from build123d import *

# Parameters (mm, degrees)
ESBO_O1_W                                            = 25
ESBO_O1_H                                            = 14
RESSALTO_EXTRUS_O1_DEPTH                             = 4
ESBO_O2_W                                            = 4
ESBO_O2_H                                            = 14
RESSALTO_EXTRUS_O2_DEPTH                             = 5
ESBO_O4_W                                            = 25
ESBO_O4_H                                            = 2
CORTE_EXTRUS_O1_DEPTH                                = 31.033314835
ESCAREADO_PARA_PARAFUSO_COM_CABE_A_ESCAR_D           = 2.4
ESCAREADO_PARA_PARAFUSO_COM_CABE_A_ESCAR_DEPTH       = 15
ESCAREADO_PARA_PARAFUSO_COM_CABE_A_ESCAR_CSINK_D     = 4.4
ESCAREADO_PARA_PARAFUSO_COM_CABE_A_ESCAR_CSINK_ANGLE = 90
ESCAREADO_PARA_PARAFUSO_COM_CABE_A_ESCAR_TIP         = 0.721032743
FILETE1_R                                            = 2
CHANFRO1_SIZE                                        = 1


with BuildPart() as part:
    # Esboço1 → Ressalto-extrusão1 (new body)
    with BuildSketch(Plane.XY):
        with Locations((12.5, 7)):
            Rectangle(ESBO_O1_W, ESBO_O1_H)
    extrude(amount=RESSALTO_EXTRUS_O1_DEPTH)

    # Esboço2 → Ressalto-extrusão2 (add)
    with BuildSketch(Plane.XY.offset(4)):
        with Locations((23, 7)):
            Rectangle(ESBO_O2_W, ESBO_O2_H)
    extrude(amount=RESSALTO_EXTRUS_O2_DEPTH)

    # Esboço4 → Corte-extrusão1 (cut, through all)
    with BuildSketch(Plane.XY.offset(9)):
        with Locations((12.5, 13)):
            Rectangle(ESBO_O4_W, ESBO_O4_H)
        with Locations((12.5, 1)):
            Rectangle(ESBO_O4_W, ESBO_O4_H)
    extrude(amount=-CORTE_EXTRUS_O1_DEPTH, mode=Mode.SUBTRACT)

    # Escareado para parafuso com cabeça escareada chata de M21
    with Locations(Plane(origin=(21, 10, 7), x_dir=(0, -1, 0), z_dir=(-1, 0, 0))):
        with Locations((0, 0), (6, 0)):
            CounterSinkHole(ESCAREADO_PARA_PARAFUSO_COM_CABE_A_ESCAR_D / 2, ESCAREADO_PARA_PARAFUSO_COM_CABE_A_ESCAR_CSINK_D / 2, depth=ESCAREADO_PARA_PARAFUSO_COM_CABE_A_ESCAR_DEPTH, counter_sink_angle=ESCAREADO_PARA_PARAFUSO_COM_CABE_A_ESCAR_CSINK_ANGLE)
            with Locations((0, 0, -(ESCAREADO_PARA_PARAFUSO_COM_CABE_A_ESCAR_DEPTH + ESCAREADO_PARA_PARAFUSO_COM_CABE_A_ESCAR_TIP / 2))):  # 118° drill point
                Cone(0, ESCAREADO_PARA_PARAFUSO_COM_CABE_A_ESCAR_D / 2, ESCAREADO_PARA_PARAFUSO_COM_CABE_A_ESCAR_TIP, mode=Mode.SUBTRACT)

    # Filete1
    filete1_edges = [part.edges().sort_by_distance(p)[0] for p in [
        (25, 7, 0),
    ]]
    fillet(filete1_edges, radius=FILETE1_R)

    # Chanfro1
    # the kernel refuses this chamfer: 1 mm, written as the material it takes off along each edge
    with BuildSketch(Plane(origin=(0, 14.571682988, 4), x_dir=(-0.027495876610586365, 0, -0.9996219169112968), z_dir=(0, -1, 0))) as chanfro1_piece_1:
        Polygon((CHANFRO1_SIZE * 0.999621916911, CHANFRO1_SIZE * 0.0274958766106), (-CHANFRO1_SIZE * 0.0274958766106, CHANFRO1_SIZE * 0.999621916911), (0, 0), align=None)
    extrude(amount=15.143365976, mode=Mode.SUBTRACT)
    with BuildSketch(Plane(origin=(21, 12, 4), x_dir=(0, 0.02749587661058735, -0.9996219169112968), z_dir=(-1, 0, 0))) as chanfro1_piece_2:
        Polygon((CHANFRO1_SIZE * 0.999621916911, CHANFRO1_SIZE * 0.0274958766106), (-CHANFRO1_SIZE * 0.0274958766106, CHANFRO1_SIZE * 0.999621916911), (0, 0), align=None)
    extrude(amount=23.571682988, mode=Mode.SUBTRACT)
    with BuildSketch(Plane(origin=(21, 12, 5.344832151), x_dir=(0.9996219169112968, 0.027495876610585647, 0), z_dir=(0, 0, 1)), Plane(origin=(21, 2, 11.571682988), x_dir=(0.9996219169112968, -0.027495876610586726, 0), z_dir=(0, 0, -1))) as chanfro1_piece_3:
        Polygon((CHANFRO1_SIZE * 0.999621916911, -CHANFRO1_SIZE * 0.0274958766106), (-CHANFRO1_SIZE * 0.0274958766106, -CHANFRO1_SIZE * 0.999621916911), (0, 0), align=None)
    extrude(amount=6.226850837, mode=Mode.SUBTRACT)
    with BuildSketch(Plane(origin=(-2.571682988, 2, 4), x_dir=(0, 0.9996219169112968, 0.027495876610586487), z_dir=(1, 0, 0))) as chanfro1_piece_4:
        Polygon((CHANFRO1_SIZE * 0.999621916911, -CHANFRO1_SIZE * 0.0274958766106), (-CHANFRO1_SIZE * 0.0274958766106, -CHANFRO1_SIZE * 0.999621916911), (0, 0), align=None)
    extrude(amount=23.571682988, mode=Mode.SUBTRACT)
    with BuildSketch(Plane(origin=(21, 2, 8.655167849), x_dir=(-0.027495876610585623, 0.9996219169112968, 0), z_dir=(0, 0, -1))) as chanfro1_piece_5:
        Polygon((CHANFRO1_SIZE * 0.999621916911, CHANFRO1_SIZE * 0.0274958766106), (-CHANFRO1_SIZE * 0.0274958766106, CHANFRO1_SIZE * 0.999621916911), (0, 0), align=None)
    extrude(amount=4.655167849, mode=Mode.SUBTRACT)
    with BuildSketch(Plane(origin=(21, 12, 4), x_dir=(0.9996219169112968, 0.027495876610585647, 0), z_dir=(0, 0, 1))) as chanfro1_piece_6:
        Polygon((CHANFRO1_SIZE * 0.999621916911, -CHANFRO1_SIZE * 0.0274958766106), (-CHANFRO1_SIZE * 0.0274958766106, -CHANFRO1_SIZE * 0.999621916911), (0, 0), align=None)
    extrude(amount=4.655167849, mode=Mode.SUBTRACT)
    with BuildSketch(Plane(origin=(23.571682988, 12, 4), x_dir=(0, 0.027495876610585623, -0.9996219169112968), z_dir=(-1, 0, 0))) as chanfro1_piece_7a_section:
        Polygon((CHANFRO1_SIZE * 0.999621916911, CHANFRO1_SIZE * 0.0274958766106), (-CHANFRO1_SIZE * 0.0274958766106, CHANFRO1_SIZE * 0.999621916911), (0, 0), align=None)
    chanfro1_piece_7a = extrude(amount=26.143365976, mode=Mode.PRIVATE)
    chanfro1_piece_7a = split(chanfro1_piece_7a, bisect_by=Plane(origin=(21, 11.670206373, 3.670206373), z_dir=(1, 0, 0)), keep=Keep.TOP, mode=Mode.PRIVATE)
    with BuildSketch(Plane(origin=(21, 12, 1.428317012), x_dir=(0.9996219169112968, 0.027495876610585647, 0), z_dir=(0, 0, 1))) as chanfro1_piece_7b_section:
        Polygon((CHANFRO1_SIZE * 0.999621916911, -CHANFRO1_SIZE * 0.0274958766106), (-CHANFRO1_SIZE * 0.0274958766106, -CHANFRO1_SIZE * 0.999621916911), (0, 0), align=None)
    chanfro1_piece_7b = extrude(amount=7.226850837, mode=Mode.PRIVATE)
    chanfro1_piece_7b = split(chanfro1_piece_7b, bisect_by=Plane(origin=(21.329793627, 11.670206373, 4), z_dir=(0, 0, -1)), keep=Keep.TOP, mode=Mode.PRIVATE)
    chanfro1_piece_7 = chanfro1_piece_7a & chanfro1_piece_7b
    add(chanfro1_piece_7, mode=Mode.SUBTRACT)
    with BuildSketch(Plane(origin=(-2.571682988, 2, 4), x_dir=(0, 0.9996219169112968, 0.027495876610586487), z_dir=(1, 0, 0))) as chanfro1_piece_8a_section:
        Polygon((CHANFRO1_SIZE * 0.999621916911, -CHANFRO1_SIZE * 0.0274958766106), (-CHANFRO1_SIZE * 0.0274958766106, -CHANFRO1_SIZE * 0.999621916911), (0, 0), align=None)
    chanfro1_piece_8a = extrude(amount=26.143365976, mode=Mode.PRIVATE)
    chanfro1_piece_8a = split(chanfro1_piece_8a, bisect_by=Plane(origin=(21, 2.329793627, 3.670206373), z_dir=(1, 0, 0)), keep=Keep.TOP, mode=Mode.PRIVATE)
    with BuildSketch(Plane(origin=(21, 2, 8.655167849), x_dir=(-0.027495876610585623, 0.9996219169112968, 0), z_dir=(0, 0, -1))) as chanfro1_piece_8b_section:
        Polygon((CHANFRO1_SIZE * 0.999621916911, CHANFRO1_SIZE * 0.0274958766106), (-CHANFRO1_SIZE * 0.0274958766106, CHANFRO1_SIZE * 0.999621916911), (0, 0), align=None)
    chanfro1_piece_8b = extrude(amount=7.226850837, mode=Mode.PRIVATE)
    chanfro1_piece_8b = split(chanfro1_piece_8b, bisect_by=Plane(origin=(21.329793627, 2.329793627, 4), z_dir=(0, 0, -1)), keep=Keep.TOP, mode=Mode.PRIVATE)
    chanfro1_piece_8 = chanfro1_piece_8a & chanfro1_piece_8b
    add(chanfro1_piece_8, mode=Mode.SUBTRACT)


solid = part.part
Could you check a few things on this model? Use its own coordinates, in mm. A direction names the side the tool comes from. Coordinates: 2 decimals unless noted, no trailing zeros. Order: outer loops, then holes, each group sorted by start corner. A loop starts at its lowest first (then second) coordinate and runs counter-clockwise, first axis right, second up. Notation, with made-up numbers: (45.25, -34.5) -> (67.25, -34.5) arc R18 cw to (67.25, -22.5) -> close; hole circle Ø6 at (17.5, -0.5). An arc over 180 degrees is marked (long way). One line per item, written item: value. Start each with the question number.
1) If I drill on L1, parallel to Y at x = 23.7, z = 7; L2, parallel to Z at x = 4.5, y = 10.75; L3, parallel to Z at x = 23.95, y = 10, over which ranges is the centre line in solid material (lowest first)? Write a range as [from, to].
2) We'd pull the mould along Z, two halves only. Please class faces 1 (the flat face through (23, 7, 9)), 2 (the flat face through (11, 7, 0)), 3 (the cylindrical face through (23.52, 3.84, 8.19)): +Z half, -Z half, draft (parallel to the pull), parting line (faces both ways), or undercut.
3) Imagine slicing it at A-A on z = 7. List the corners of the cut face in (x, y) for me, plus the area to 3 significant figures.
4) Which directions (+Z, -Z, +X, -X, +Y, -Y) give clear straight access to the entire face, cutting with the end or side of a thin tool? Please do faces 4 (the flat face through (21, 7, 6)), 5 (the flat face through (11.2, 11.5, 3.5)), 6 (the flat face through (21.6, 2.4, 6)).
5) I'm going to push flat-ended pins straight in: pin 1 (3 mm diameter, centred on y = 10, z = 7, fed in from -X); pin 2 (1 mm diameter, centred on x = 16.5, y = 11, fed in from +Z); pin 3 (2.5 mm diameter, centred on y = 8, z = 5.5, fed in from -X). Where does each tip first touch, or does it pass through?
6) Imagine slicing it at C-C on x = 2. List the corners of the cut face in (y, z) for me.
7) Imagine slicing it at D-D on z = 0.5. List the corners of the cut face in (x, y) for me.
8) Imagine slicing it at B-B on y = 4. List the corners of the cut face in (x, z) for me.
Answer list:
1. L1: y = [2, 2.8], [5.2, 8.8], [11.2, 12]
1. L2: z = [0, 4]
1. L3: z = [0.24, 5.8], [8.2, 9]
2. face 1: +Z half
2. face 2: -Z half
2. face 3: undercut
3. outline: (21, 6.2) -> (22, 5.2) -> (25, 5.2) -> (25, 8.8) -> (22, 8.8) -> (21, 7.8) -> close; (21.6, 2.4) -> (22, 2) -> (25, 2) -> (25, 2.8) -> (22, 2.8) -> close; (21.6, 11.6) -> (22, 11.2) -> (25, 11.2) -> (25, 12) -> (22, 12) -> close
3. area: 18.5 mm2
4. face 4: +Z, -X, +Y, -Y
4. face 5: +Z, -X, +Y
4. face 6: +Z, -X, -Y
5. pin 1: stops at x = 21.7
5. pin 2: stops at z = 4
5. pin 3: stops at x = 21
6. outline: (2, 0) -> (12, 0) -> (12, 3) -> (11, 4) -> (3, 4) -> (2, 3) -> close
7. outline: (0, 2) -> (24.32, 2) -> (24.32, 12) -> (0, 12) -> close
8. outline: (0, 0) -> (23, 0) arc R2 ccw to (25, 2) -> (25, 5.8) -> (22, 5.8) -> (21, 4.8) -> (21, 4) -> (1, 4) -> (0, 3) -> close; (21.2, 9) -> (22, 8.2) -> (25, 8.2) -> (25, 9) -> close
